Source: CAD feature listing. Evaluate the final solid. Frame: model axes, mm. A direction names the side the tool comes from. Round coordinates to 2 decimals unless told otherwise and drop trailing zeros. Loops run counter-clockwise (first coordinate to the right, second up) from the corner with the lowest first, then second, coordinate; pieces in that order, holes last. Notation, with made-up numbers: (64, 73.25) - (95, 73.25) arc R10 cw to (95, 86.25) - close; hole circle Ø11 at (43, -7). An arc over 180 degrees is marked (long way). One line per question, with ' | ' between items.
from build123d import *

# Parameters (mm, degrees)
SKETCH1_R           = 1.524
BOSS_EXTRUDE1_DEPTH = 3.048


with BuildPart() as part:
    # Sketch1 → Boss-Extrude1 (new body)
    with BuildSketch(Plane(origin=(0, 0, 0), x_dir=(1, 0, 0), z_dir=(0, 1, 0))):
        with BuildLine():
            Line((4.120039677, 7.385454502), (4.120039677, -20.735478746))
            ThreePointArc((4.120039677, -20.735478746), (-0.490464098, -25.345982522), (-5.100967874, -20.735478746))
            Line((-5.100967874, -20.735478746), (-5.100967874, 7.385454502))
            ThreePointArc((-5.100967874, 7.385454502), (-5.569137189, 10.778713446), (-7.306945844, 13.730561993))
            ThreePointArc((-7.306945844, 13.730561993), (-0.490464096, 28.96950355), (6.326017651, 13.730561993))
            ThreePointArc((6.326017651, 13.730561993), (4.687262198, 10.744276018), (4.120039677, 7.385454502))
        make_face()
        with Locations(Location((-0.490464098, -20.735478746, 0), (0, 0, 90))):
            Circle(SKETCH1_R, mode=Mode.SUBTRACT)
        with Locations(Location((-0.490464096, 19.82550355, 0), (0, 0, 90))):
            Circle(SKETCH1_R, mode=Mode.SUBTRACT)
        with BuildLine():
            Line((-1.643126624, 8.246871525), (-1.643126624, 2.47327546))
            ThreePointArc((-1.643126624, 2.47327546), (-0.49050068, 1.320649517), (0.662125264, 2.47327546))
            Line((0.662125264, 2.47327546), (0.662125264, 8.246871525))
            ThreePointArc((0.662125264, 8.246871525), (-0.49050068, 9.399497469), (-1.643126624, 8.246871525))
        make_face(mode=Mode.SUBTRACT)
    extrude(amount=BOSS_EXTRUDE1_DEPTH)


solid = part.part
1. Mould query, pull axis X, two halves, no side actions, for faces 4 (the cylindrical face through (4.703, 1.503, -10.789)), 5 (the cylindrical face through (-5.553, 1.503, -10.733)), 6 (the cylindrical face through (-0.557, 1.503, -18.303)). Classes: released by +X, released by -X, zero draft, split by the parting line, or undercut.
Worked out:
face 4: released by +X | face 5: released by -X | face 6: undercut
2. Section query A-A, the plane z = -4. Return loops of the section in (x, y), plus the area to 3 significant figures.
Worked out:
outline: (-5.1, 0) - (-1.64, 0) - (-1.64, 3.05) - (-5.1, 3.05) - close; (0.66, 0) - (4.12, 0) - (4.12, 3.05) - (0.66, 3.05) - close | area: 21.1 mm2
3. Section query C-C, the plane z = -20.5. Return loops of the section in (x, y).
Worked out:
outline: (-9.61, 0) - (-1.86, 0) - (-1.86, 3.05) - (-9.61, 3.05) - close; (0.88, 0) - (8.63, 0) - (8.63, 3.05) - (0.88, 3.05) - close
4. Section query D-D, the plane x = 2. Return loops of the section in (y, z), plus the area to 3 significant figures.
Worked out:
outline: (0, -28.62) - (3.05, -28.62) - (3.05, 24.62) - (0, 24.62) - close | area: 162 mm2
5. Section query B-B, the plane y = 1.5. Return loops of the section in (x, z).
Worked out:
outline: (-7.31, -13.73) arc R9.14 ccw (long way) to (6.33, -13.73) arc R10.23 cw to (4.12, -7.39) - (4.12, 20.74) arc R4.61 ccw to (-5.1, 20.74) - (-5.1, -7.39) arc R8.73 cw to start; hole circle Ø3.05 at (-0.49, -19.83); hole circle Ø3.05 at (-0.49, 20.74); hole (-1.64, -8.25) arc R1.15 ccw to (0.66, -8.25) - (0.66, -2.47) arc R1.15 ccw to (-1.64, -2.47) - close
6. Access query for faces 1 (the flat face through (4.12, 2, 6)), 2 (the cylindrical face through (-0.5, 1.5, -9.4)), 3 (the flat face through (-5.101, 2, 7)). Directions: +Z, -Z, +X, -X, +Y, -Y. A direction counts if a zero-diameter tool reaches every point of the face in a straight line with its end or side. Return the directions, or none.
Worked out:
face 1: +Z, +X, +Y, -Y | face 2: +Y, -Y | face 3: +Z, -X, +Y, -Y
7. Material intervals for probe 1 along X at (y, z) = (0.9, -5); probe 2 along X at (y, z) = (2.5, -19.5); probe 3 along Z at (x, y) = (-1, 1.65), sorted ascending.
Worked out:
probe 1: x = -5.1 to -1.64, 0.66 to 4.12 | probe 2: x = -9.63 to -1.98, 1 to 8.65 | probe 3: z = -28.96 to -21.26, -18.39 to -9.28, -1.44 to 19.3, 22.17 to 25.32
8. Contact query for flat-ended pins moving along their axis: P1, Ø1.8, axis at x = -0.49, z = 20.74, coming from the +Y side; P2, Ø1.5, axis at y = 2, z = 4, coming from the -X side; P3, Ø1.5, axis at y = 2, z = -5.5, coming from the +X side. Output: stop coordinate, or through.
Worked out:
P1: passes through | P2: stops at x = -5.1 | P3: stops at x = 4.12
